Verification items for the finished model (mm, model axes). A direction names the side the tool comes from. Round coordinates to 2 decimals unless told otherwise and drop trailing zeros. Loops run counter-clockwise (first coordinate to the right, second up) from the corner with the lowest first, then second, coordinate; pieces in that order, holes last. Notation, with made-up numbers: (39, 16) -> (82, 16) arc R18 cw to (82, 46) -> close; hole circle Ø4 at (18.5, 66.25). An arc over 180 degrees is marked (long way). Write item = value, one per line.
```python
from build123d import *

# Parameters (mm, degrees)
PAD_DEPTH     = 3
SKETCH001_R   = 2.75
PAD001_DEPTH  = 2
CHAMFER_SIZE2 = 1.99
CHAMFER_SIZE  = 1
SKETCH002_R   = 1.55
POCKET_DEPTH  = 5
FILLET_R      = 1.15625


with BuildPart() as part:
    # Sketch → Pad (new body)
    with BuildSketch(Plane.XY):
        Polygon((0, 0), (0, 41.625), (19.656, 41.625), (19.656, 46.25), (38.156, 46.25), (38.156, 48.563), (56.656, 48.563), (56.656, 46.25), (76.312, 46.25), (76.312, 19.656), (84.406, 19.656), (84.406, 0), align=None)
    extrude(amount=PAD_DEPTH)

    # Sketch001 (on Face14 of Pad) → Pad001 (join)
    with BuildSketch(Plane.XY.offset(3)):
        with Locations((10.657, 21.75)):
            Circle(SKETCH001_R)
        with Locations((34.938, 21.75)):
            Circle(SKETCH001_R)
    extrude(amount=PAD001_DEPTH)

    # Chamfer
    chamfer_edges = [part.edges().sort_by_distance(p)[0] for p in [
        (7.907, 21.75, 3),
        (32.188, 21.75, 3),
    ]]
    chamfer_side = part.faces().sort_by_distance((41.05483, 22.316964, 3))[0]
    chamfer(chamfer_edges, length=CHAMFER_SIZE, length2=CHAMFER_SIZE2, reference=chamfer_side)

    # Sketch002 (on Face19 of Chamfer) → Pocket (cut)
    with BuildSketch(Plane.XY.offset(5)):
        with Locations((10.657, 21.75)):
            Circle(SKETCH002_R)
        with Locations((34.938, 21.75)):
            Circle(SKETCH002_R)
    extrude(amount=-POCKET_DEPTH, mode=Mode.SUBTRACT)

    # Fillet
    fillet_edges = [part.edges().sort_by_distance(p)[0] for p in [
        (84.406, 0, 1.5),
        (84.406, 19.656, 1.5),
        (76.312, 19.656, 1.5),
        (76.312, 46.25, 1.5),
        (56.656, 46.25, 1.5),
        (56.656, 48.563, 1.5),
        (38.156, 48.563, 1.5),
        (19.656, 46.25, 1.5),
        (0, 41.625, 1.5),
        (38.156, 46.25, 1.5),
        (19.656, 41.625, 1.5),
        (0, 0, 1.5),
    ]]
    fillet(fillet_edges, radius=FILLET_R)


solid = part.part
```
(1) Sectioned sample at C-C, the plane z = 4.15. Record the cut outline in (x, y), and give its area (3 significant figures).
Filled sheet:
outline = circle Ø6.34 at (10.66, 21.75); circle Ø6.34 at (34.94, 21.75); hole circle Ø3.1 at (10.66, 21.75); hole circle Ø3.1 at (34.94, 21.75)
area = 48.1 mm2
(2) Go/stop test with flat-tipped pins: pin 1 Ø1 at (y, z) = (36.5, 3) entering from +X; pin 2 Ø0.9 at (x, z) = (79.5, 2) entering from +Y; pin 3 Ø2.5 at (x, z) = (70.5, 1.5) entering from +Y. Record where each tip stops, or that it passes through.
Filled sheet:
pin_1 = 76.31
pin_2 = 19.66
pin_3 = 46.25
(3) Sectioned sample at A-A, the plane y = 21.75. Count the separate pieces of the cut face and the enclosed holes in it, and give its area (3 significant figures).
Filled sheet:
separate_pieces = 3
enclosed_holes = 0
area = 224 mm2
(4) Draft check along X on faces 4 (the face through (35.77, 23.06, 2.54)), 5 (the face through (47, 48.563, 1)), 6 (the face through (10.455, 23.287, 2.535)), 7 (the face through (76.312, 33, 1)). Enter one of: released by +X, released by -X, zero draft, split by the parting line, or undercut.
Filled sheet:
face_4 = undercut
face_5 = zero draft
face_6 = undercut
face_7 = released by +X
(5) Material ranges on probe 1 along Z at (x, y) = (48.5, 39); probe 2 along Y at (x, z) = (63.5, 2.15); probe 3 along X at (y, z) = (38.5, 1.15), recorded low to high. Write a range as from..to.
Filled sheet:
probe_1 = 0..3
probe_2 = 0..46.25
probe_3 = 0..76.31
(6) Sectioned sample at B-B, the plane x = 70. Record the cut outline in (y, z).
Filled sheet:
outline = (0, 0) -> (46.25, 0) -> (46.25, 3) -> (0, 3) -> close
(7) Sectioned sample at D-D, the plane y = 34. Record the cut outline in (x, z), and give its area (3 significant figures).
Filled sheet:
outline = (0, 0) -> (76.31, 0) -> (76.31, 3) -> (0, 3) -> close
area = 229 mm2
(8) Set-up check for faces 1 (the face through (19.656, 44, 1)), 2 (the face through (80, 19.656, 1)), 3 (the face through (12.5, 21.8, 5)): record each of +Z, -Z, +X, -X, +Y, -Y from which the full face is reachable in a straight line by a thin tool's end or side.
Filled sheet:
face_1 = +Z, -Z, -X, +Y
face_2 = +Z, -Z, +X, +Y
face_3 = +Z, +X, -X, +Y, -Y
